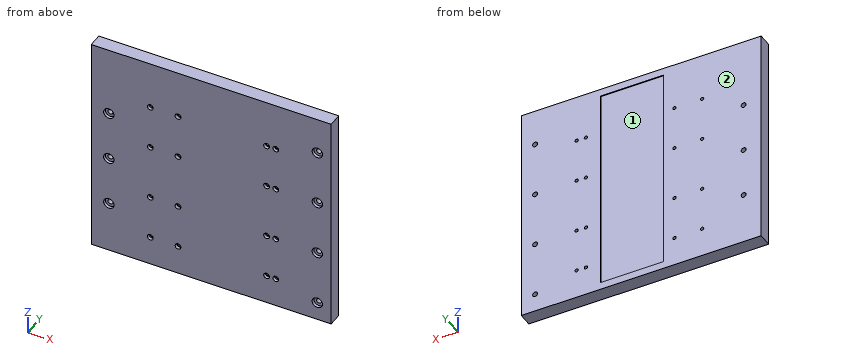
```python
from build123d import *

# Parameters (mm, degrees)
SKETCH1_W                                            = 330.2
SKETCH1_H                                            = 304.8
BOSS_EXTRUDE1_DEPTH                                  = 19.05
SKETCH2_W                                            = 86.36
SKETCH2_H                                            = 284.48
CUT_EXTRUDE1_DEPTH                                   = 1.016
CBORE_FOR_8_SOCKET_HEAD_CAP_SCREW1_D                 = 4.4958
CBORE_FOR_8_SOCKET_HEAD_CAP_SCREW1_CBORE_D           = 7.9375
CBORE_FOR_8_SOCKET_HEAD_CAP_SCREW1_CBORE_DEPTH       = 4.1656
CBORE_FOR_1_4_BINDING_HEAD_MACHINE_SCREW_D           = 6.7564
CBORE_FOR_1_4_BINDING_HEAD_MACHINE_SCREW_CBORE_D     = 14.2875
CBORE_FOR_1_4_BINDING_HEAD_MACHINE_SCREW_CBORE_DEPTH = 4.191


with BuildPart() as part:
    # Sketch1 → Boss-Extrude1 (new body)
    with BuildSketch(Plane(origin=(0, 0, 0), x_dir=(1, 0, 0), z_dir=(0, 1, 0))):
        with Locations((165.1, -152.4)):
            Rectangle(SKETCH1_W, SKETCH1_H)
    extrude(amount=BOSS_EXTRUDE1_DEPTH)

    # Sketch2 → Cut-Extrude1 (cut)
    with BuildSketch(Plane(origin=(0, 19.05, 0), x_dir=(1, 0, 0), z_dir=(0, 1, 0))):
        with Locations((177.8, -152.4)):
            Rectangle(SKETCH2_W, SKETCH2_H)
    extrude(amount=-CUT_EXTRUDE1_DEPTH, mode=Mode.SUBTRACT)

    # CBORE for #8 Socket Head Cap Screw1 (through all)
    with Locations(Plane(origin=(0, 0, 0), x_dir=(-1, 0, 0), z_dir=(0, -1, 0))):
        with Locations((-241.3, -40.64), (-254, -40.64), (-254, -101.6), (-241.3, -101.6), (-241.3, -177.8), (-254, -177.8), (-254, -238.76), (-241.3, -238.76), (-119.38, -40.64), (-81.28, -40.64), (-81.28, -101.6), (-119.38, -101.6), (-119.38, -177.8), (-81.28, -177.8), (-81.28, -238.76), (-119.38, -238.76)):
            CounterBoreHole(CBORE_FOR_8_SOCKET_HEAD_CAP_SCREW1_D / 2, CBORE_FOR_8_SOCKET_HEAD_CAP_SCREW1_CBORE_D / 2, CBORE_FOR_8_SOCKET_HEAD_CAP_SCREW1_CBORE_DEPTH)

    # CBORE for 1/4 Binding Head Machine Screw1 (through all)
    with Locations(Plane(origin=(0, 0, 0), x_dir=(-1, 0, 0), z_dir=(0, -1, 0))):
        with Locations((-311.15, -25.4), (-311.15, -101.6), (-311.15, -177.8), (-311.15, -254), (-24.13, -71.12), (-24.13, -139.7), (-24.13, -208.28)):
            CounterBoreHole(CBORE_FOR_1_4_BINDING_HEAD_MACHINE_SCREW_D / 2, CBORE_FOR_1_4_BINDING_HEAD_MACHINE_SCREW_CBORE_D / 2, CBORE_FOR_1_4_BINDING_HEAD_MACHINE_SCREW_CBORE_DEPTH)


solid = part.part
```
Here's how the part is built. I have some questions about the finished solid (model axes, mm). Face numbers are marked on the shaded views. Give positions to 0.01 mm unless a question says otherwise; leave off trailing zeros. Write each loop counter-clockwise with the first axis right and the second up, starting at its lowest first coordinate (ties: lowest second). Pieces come first, ordered by that corner, then holes. Notation, with made-up numbers: M -32,27.5 L -14,27.5 A14 ccw -14,36.5 Z; hole C 24,83 d9. An arc over 180 degrees is marked long. Put each result on its own line as item: value. Start each with the question number.
Item 1: I need wall thicknesses on L1, parallel to X at y = 1, z = 177.8; L2, parallel to Z at x = 254, y = 2; L3, parallel to X at y = 14, z = 101.6. Which ranges of each line are inside material? Lowest first, please. Write a range as from..to.
Item 2: Will this pin go through, and if not, where does the flat tip stop? pin 1 (5 mm diameter, centred on x = 254, z = 101.6, fed in from -Y).
Item 3: Thinking about a two-plate mould opening in Z: for the marked faces 1 and 2, which applies, +Z half, -Z half, draft (parallel to the pull), parting line (faces both ways), or undercut?
Item 4: If we section it at A-A, the plane x = 204: Write out the boundary of the cut face in (y, z).
Values:
1. L1: 0..77.31, 85.25..115.41, 123.35..237.33, 245.27..250.03, 257.97..304.01, 318.29..330.2
1. L2: 0..36.67, 44.61..97.63, 105.57..173.83, 181.77..234.79, 242.73..304.8
1. L3: 0..79.03, 83.53..117.13, 121.63..239.05, 243.55..251.75, 256.25..307.77, 314.53..330.2
2. pin 1: y = 4.17
3. face 1: undercut
3. face 2: draft
4. outline: M 0,0 L 19.05,0 L 19.05,10.16 L 18.03,10.16 L 18.03,294.64 L 19.05,294.64 L 19.05,304.8 L 0,304.8 Z
